Autodesk Inventor part; units mm, degrees
ref_plane "Work Plane1" through (0, -12, 0) normal (0, 1, 0) x (-1, 0, 0)
ref_plane "YZ Plane" through (0, 0, 0) normal (1, 0, 0) x (0, 1, 0)
ref_plane "XY Plane" through (0, 0, 0) normal (0, 0, 1) x (1, 0, 0)
sketch "Sketch1" plane through (0, 0, 0) normal (0, 0, 1) x (1, 0, 0)
  circle A0 centre (0, 0) radius 12
  circle A1 centre (0, 0) radius 10
  dimension "d0" = 24
  dimension "d1" = 20
extrude "Extrusion1" add sketch "Sketch1" along normal blind 500
ref_plane "Work Plane1" through (0, -12, 0) normal (0, 1, 0) x (-1, 0, 0)
sketch "Sketch2" plane through (0, -12, 0) normal (0, 1, 0) x (-1, 0, 0)
  line L0 (-136.7178, 142) -> (138.1684, 142)
  line L1 (12, 0) -> (-12, 0)
  point P0 (0, 0)
  dimension "d4" = 142
bend part "Bend Part1" radius 25.4 angle 40 line through (136.7178, -12, 142) along (-1, 0, 0) centre toward (0, 1, 0) moving side (0, 0, -1) both sides no
properties part number "Sit Link 2"
Here's how the part is built. I have some questions about the finished solid (model axes, mm). A direction names the side the tool comes from. Coordinates: 2 decimals unless noted, no trailing zeros. Order: outer loops, then holes, each group sorted by start corner. A loop starts at its lowest first (then second) coordinate and runs counter-clockwise, first axis right, second up. Notation, with made-up numbers: M 3.5,13 L 62.5,13 A6 ccw 62.5,22 Z; hole C 4,-39 d9. An arc over 180 degrees is marked long. Answer as a JSON object with one key per item and string values. Group by question number.
(1) I need wall thicknesses on probe 1 along X at (y, z) = (0, 354); probe 2 along Y at (x, z) = (-7.75, 108.5). Which ranges of each line are inside material? Lowest first, please.
(2) Suppose I cut it at A-A, the plane x = 0. Please give me the cut outline in (y, z), then the cut area to 3 significant figures.
(3) If we mould it in two halves opening along X, with no side actions, what happens to faces 3 (the face through (-11.99, -0.53, 318.49)), 4 (the face through (9.538, 41.332, 83.192)), 5 (the face through (-2.723, 90.546, 44.513))? For each: released by +X, released by -X, zero draft, split by the parting line, or undercut.
(4) For pin 1 (3 mm diameter, centred on x = -5.5, z = 164, fed in from +Y); pin 2 (1.5 mm diameter, centred on x = -2.5, z = 340, fed in from +Y); pin 3 (1 mm diameter, centred on x = 5.5, y = 44.5, fed in from -Z), each with a flat end and sliding along its axis, tell me the tip position at first contact or that it passes through.
(5) Which directions (+Z, -Z, +X, -X, +Y, -Y) give clear straight access to the entire face, cutting with the end or side of a thin tool? Please do faces 1 (the face through (11.446, 40.872, 82.806)), 2 (the face through (-2.17, 9.76, 318.49)).
Values found:
{
 "1": {"probe 1": "x = -12 to -10, 10 to 12", "probe 2": "y = 12.06 to 15.77, 32.27 to 35.98"},
 "2": {"outline": "M -12,142 A25.4 ccw -6.06,125.67 L 73.82,30.48 L 75.35,31.76 L -4.53,126.96 A23.4 cw -10,142 L -10,500 L -12,500 Z; M 10,142 A3.4 ccw 10.8,139.81 L 90.67,44.62 L 92.21,45.91 L 12.33,141.1 A1.4 cw 12,142 L 12,500 L 10,500 Z", "area": "1,970 mm^2"},
 "3": {"face 3": "split by the parting line", "face 4": "undercut", "face 5": "zero draft"},
 "4": {"pin 1": "stops at y = 11.31", "pin 2": "stops at y = 11.87", "pin 3": "stops at z = 66.79"},
 "5": {"face 1": "none", "face 2": "+Z"}
}
